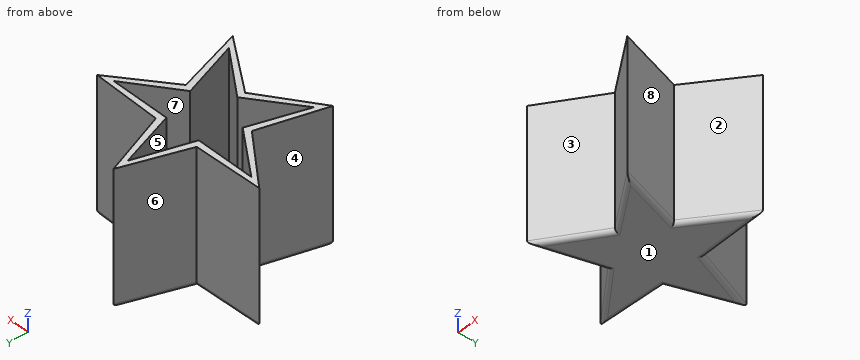
```python
from build123d import *

# Parameters (mm, degrees)
F1_DEPTH = 50.8
F3_DEPTH = 10.16
F4_R     = 3.175


with BuildPart() as f1:
    # F0 (on Top) → F1 (new body, symmetric)
    with BuildSketch(Plane.XY):
        Polygon((13.549365, 18.649101), (0, 60.501583), (-13.549365, 18.649101), (-57.540424, 18.696017), (-21.923333, -7.123323), (-35.561938, -48.946809), (0, -23.051556), (35.561938, -48.946809), (21.923333, -7.123323), (57.540424, 18.696017), align=None)
        Polygon((67.841942, 22.043183), (17.062389, 23.484363), (0, 71.333239), (-17.062389, 23.484363), (-67.841942, 22.043183), (-27.607525, -8.970229), (-41.928626, -57.709802), (0, -29.028269), (41.928626, -57.709802), (27.607525, -8.970229), align=None)
        Polygon((-13.549365, 18.649101), (0, 60.501583), (13.549365, 18.649101), (57.540424, 18.696017), (21.923333, -7.123323), (35.561938, -48.946809), (0, -23.051556), (-35.561938, -48.946809), (-21.923333, -7.123323), (-57.540424, 18.696017), align=None, mode=Mode.SUBTRACT)
    extrude(amount=F1_DEPTH, both=True)

    # F2 (on face) → F3 (join)
    with BuildSketch(Plane(origin=(0, 0, -50.8), x_dir=(1, 0, 0), z_dir=(0, 0, -1))):
        Polygon((0, 23.051556), (-35.561938, 48.946809), (-21.923333, 7.123323), (-57.540424, -18.696017), (-13.549365, -18.649101), (0, -60.501583), (13.549365, -18.649101), (57.540424, -18.696017), (21.923333, 7.123323), (35.561938, 48.946809), align=None)
    extrude(amount=-F3_DEPTH)

    # F4
    f4_edges = [f1.edges().sort_by_distance(p)[0] for p in [
        (42.452165, 22.763773, -50.8),
        (8.531194, 47.408801, -50.8),
        (-8.531194, 47.408801, -50.8),
        (-42.452165, 22.763773, -50.8),
        (-47.724733, 6.536477, -50.8),
        (-34.768075, -33.340016, -50.8),
        (-20.964313, -43.369036, -50.8),
        (20.964313, -43.369036, -50.8),
        (34.768075, -33.340016, -50.8),
        (47.724733, 6.536477, -50.8),
    ]]
    fillet(f4_edges, radius=F4_R)


solid = f1.part
```
Geometry check sheet. Reference: the model listing, model coordinates, mm. Face numbers are marked on the shaded views. A direction names the side the tool comes from. Coordinates: 2 decimals unless noted, no trailing zeros. Order: outer loops, then holes, each group sorted by start corner. A loop starts at its lowest first (then second) coordinate and runs counter-clockwise, first axis right, second up.
Q1. Thickness scan on probe 1 along X at (y, z) = (-33.5, -38.5); probe 2 along X at (y, z) = (-38.5, 11); probe 3 along X at (y, z) = (18, 22.5). Record the ranges inside material, lowest first.
Reply:
probe 1: x = -34.82 to -30.52, -14.35 to -6.54, 6.54 to 14.35, 30.52 to 34.82
probe 2: x = -36.28 to -32.16, -21.22 to -13.85, 13.85 to 21.22, 32.16 to 36.28
probe 3: x = -62.6 to -56.58, 56.58 to 62.6
Q2. Tool access check on the marked faces 1, 2, 3, 4 and 5. Record the directions out of +Z, -Z, +X, -X, +Y, -Y that give a thin tool (end or side, any length) a straight path to the whole face; none if there is none.
Reply:
face 1: -Z, +X, -X, +Y, -Y
face 2: +Z, -Z, +X
face 3: +Z, -Z, -Y
face 4: +Z, -Z, -X
face 5: +Z
Q3. Depth check by flat-ended pin: pin 1 Ø1 at (x, y) = (26, 2.5) entering from +Z; pin 2 Ø3 at (x, z) = (-29, 13.5) entering from +Y; pin 3 Ø3 at (y, z) = (-7, -14) entering from -X; pin 4 Ø5 at (x, y) = (3.5, 54) entering from -Z. Enter the tip coordinate at first touch or a pass-through.
Reply:
pin 1: stops at z = -40.64
pin 2: stops at y = 23.19
pin 3: stops at x = -32.11
pin 4: stops at z = -50.8
Q4. Sectioned sample at A-A on z = -1. Record the cut outline in (x, y).
Reply:
outline: (-67.84, 22.04) - (-27.61, -8.97) - (-41.93, -57.71) - (0, -29.03) - (41.93, -57.71) - (27.61, -8.97) - (67.84, 22.04) - (17.06, 23.48) - (0, 71.33) - (-17.06, 23.48) - close; hole (-57.54, 18.7) - (-21.92, -7.12) - (-35.56, -48.95) - (0, -23.05) - (35.56, -48.95) - (21.92, -7.12) - (57.54, 18.7) - (13.55, 18.65) - (0, 60.5) - (-13.55, 18.65) - close
Q5. Draft check along X on the marked faces 6, 7 and 8. Enter one of: released by +X, released by -X, zero draft, split by the parting line, or undercut.
Reply:
face 6: released by -X
face 7: undercut
face 8: released by +X
